Verification items for this drawing (mm, ordinates from the low corner). A direction names the side the tool comes from. Give positions to 0.01 mm unless a question says otherwise; leave off trailing zeros. Order: outer loops, then holes, each group sorted by start corner. A loop starts at its lowest first (then second) coordinate and runs counter-clockwise, first axis right, second up.
(1) Sectioned sample at D-D on z = 3.5. Record the cut outline in (x, y), plus the area to 3 significant figures.
(2) Sectioned sample at B-B on x = 3. Record the cut outline in (y, z), plus the area to 3 significant figures.
(3) Sectioned sample at A-A on y = 1.75. Record the cut outline in (x, z).
(4) Sectioned sample at C-C on y = 6. Record the cut outline in (x, z).
(5) Gauge pin test, flat ends, axial feed: pin 1 (1.5 mm diameter, centred on y = 7.5, z = 2.5, fed in from -X); pin 2 (0.8 mm diameter, centred on x = 5.5, y = 1, fed in from +Z); pin 3 (3 mm diameter, centred on x = 1, y = 1, fed in from -Z). Record the tip position at first contact, or that the pin passes through.
(6) Access from +Z, -Z, +X, -X, +Y, -Y to the whole of each face (thin tool, end or side, straight path). Record for the marked faces 1, 2, 3 and 4.
(7) Scan lines: L1, parallel to Z at x = 1.15, y = 7; L2, parallel to Y at x = 2.45, z = 0.7; L3, parallel to Y at x = 2.8, z = 3.95. Record each from-to range of solid material in increasing order.
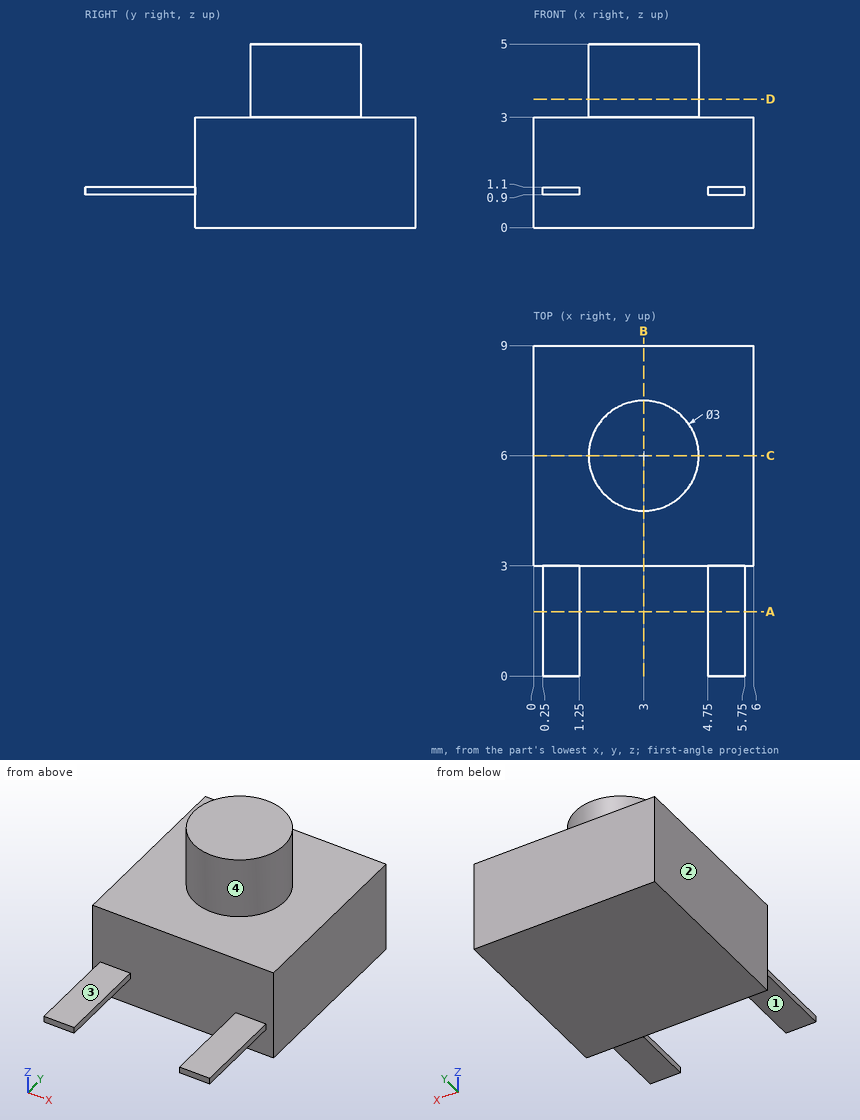
Ans:
1. outline: circle Ø3 at (3, 6)
1. area: 7.07 mm2
2. outline: (3, 0) - (9, 0) - (9, 3) - (7.5, 3) - (7.5, 5) - (4.5, 5) - (4.5, 3) - (3, 3) - close
2. area: 24.0 mm2
3. outline: (0.25, 0.9) - (1.25, 0.9) - (1.25, 1.1) - (0.25, 1.1) - close; (4.75, 0.9) - (5.75, 0.9) - (5.75, 1.1) - (4.75, 1.1) - close
4. outline: (0, 0) - (6, 0) - (6, 3) - (4.5, 3) - (4.5, 5) - (1.5, 5) - (1.5, 3) - (0, 3) - close
5. pin 1: stops at x = 0
5. pin 2: stops at z = 1.1
5. pin 3: stops at z = 0.9
6. face 1: -Z, +X, -X, -Y
6. face 2: +Z, -Z, -X, +Y, -Y
6. face 3: +Z, +X, -X, -Y
6. face 4: +Z
7. L1: z = 0 to 3
7. L2: y = 3 to 9
7. L3: y = 4.51 to 7.49
